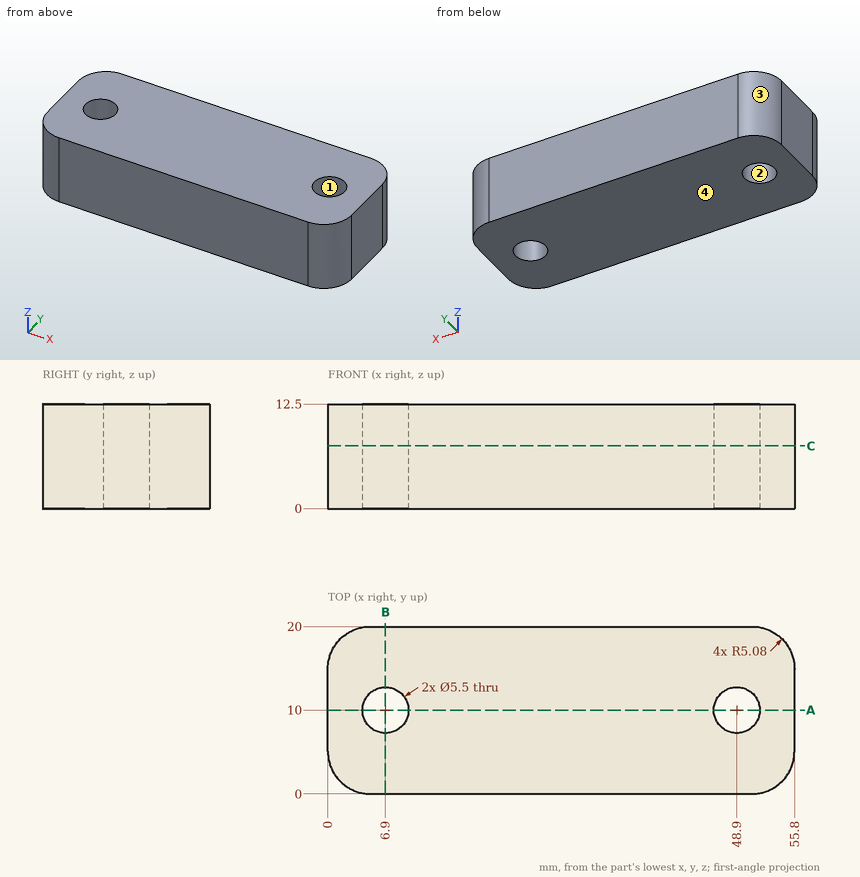
Print and shaded views of the part. All mm, measured from the part's lowest x, y and z. Coordinates: 2 decimals unless noted, no trailing zeros. Loops run counter-clockwise (first coordinate to the right, second up) from the corner with the lowest first, then second, coordinate; pieces in that order, holes last. Notation, with made-up numbers: (13.25, 74.25) - (72.25, 74.25) arc R21 cw to (72.25, 88.25) - close; hole circle Ø3 at (-35, -7.75). An arc over 180 degrees is marked (long way). Write item = value, one per line. Start each with the question number.
Item 1: Wall check: L1, parallel to Y at x = 6.9, z = 3.75; L2, parallel to X at y = 11, z = 11; L3, parallel to Y at x = 8.5, z = 2.75. Give the ranges that are in metal, low to high. Write a range as from..to.
Item 2: Cut at B-B, the plane x = 6.9. Give the cut face in (y, z).
Item 3: Cut at C-C, the plane z = 7.5. Give the cut face in (x, y), and give its area (3 significant figures).
Item 4: Mould opens along X. For the marked faces 1, 2, 3 and 4 say: released by +X, released by -X, zero draft, split by the parting line, or undercut.
Item 5: Cut at A-A, the plane y = 10. Give the cut face in (x, z), and give its area (3 significant figures).
Item 6: Flat gauge pin, fed straight in: pin 1 Ø5 at (y, z) = (2.5, 9) entering from +X. Where does the tip first touch, or does it go through?
The answers:
q1.L1 = 0..7.25, 12.75..20
q1.L2 = 0..4.34, 9.46..46.34, 51.46..55.8
q1.L3 = 0..7.76, 12.24..20
q2.outline = (0, 0) - (7.25, 0) - (7.25, 12.5) - (0, 12.5) - close; (12.75, 0) - (20, 0) - (20, 12.5) - (12.75, 12.5) - close
q3.outline = (0, 5.08) arc R5.08 ccw to (5.08, 0) - (50.72, 0) arc R5.08 ccw to (55.8, 5.08) - (55.8, 14.92) arc R5.08 ccw to (50.72, 20) - (5.08, 20) arc R5.08 ccw to (0, 14.92) - close; hole circle Ø5.5 at (6.9, 10); hole circle Ø5.5 at (48.9, 10)
q3.area = 1,050 mm2
q4.face_1 = undercut
q4.face_2 = undercut
q4.face_3 = released by -X
q4.face_4 = zero draft
q5.outline = (0, 0) - (4.15, 0) - (4.15, 12.5) - (0, 12.5) - close; (9.65, 0) - (46.15, 0) - (46.15, 12.5) - (9.65, 12.5) - close; (51.65, 0) - (55.8, 0) - (55.8, 12.5) - (51.65, 12.5) - close
q5.area = 560 mm2
q6.pin_1 = 55.8
